```python
from build123d import *

# Parameters (mm, degrees)
SKETCH1_R               = 5.053
BASENUT_DEPTH           = 10.8
ENDCHAMFER_SIZE         = 0.947
ENDCHAMFER_SIZE2        = 0.546750705
ENDCHAMFER_PART_2_SIZE  = 0.947
ENDCHAMFER_PART_2_SIZE2 = 0.546750705


with BuildPart() as part:
    # Sketch1 → BaseNut (new body)
    with BuildSketch(Plane.XY):
        Polygon((10.392304845, 0), (5.196152423, 9), (-5.196152423, 9), (-10.392304845, 0), (-5.196152423, -9), (5.196152423, -9), align=None)
        Circle(SKETCH1_R, mode=Mode.SUBTRACT)
    extrude(amount=-BASENUT_DEPTH)

    # Sketch2 → Double-Chamfer (revolve, cut)
    with BuildSketch(Plane(origin=(0, 0, 0), x_dir=(1, 0, 0), z_dir=(0, 1, 0))):
        Polygon((-10.392304845, 10.8), (-8.625, 10.8), (-10.392304845, 9.779646072), align=None)
        Polygon((-10.392304845, 1.020353928), (-10.392304845, 0), (-8.625, 0), align=None)
    revolve(axis=Axis((0, 0, -3.375940562), (0, 0, 1)), mode=Mode.SUBTRACT)

    # EndChamfer
    endchamfer_edges = [part.edges().sort_by_distance(p)[0] for p in [
        (-5.053, 0, -10.8),
    ]]
    endchamfer_side = [part.faces().sort_by_distance(p)[0] for p in [
        (-5.053, 0, -5.4),
    ]]
    chamfer(endchamfer_edges, length=ENDCHAMFER_SIZE, length2=ENDCHAMFER_SIZE2, reference=endchamfer_side[0])

    # EndChamfer part 2
    endchamfer_part_2_edges = [part.edges().sort_by_distance(p)[0] for p in [
        (-5.053, 0, 0),
    ]]
    endchamfer_part_2_side = [part.faces().sort_by_distance(p)[0] for p in [
        (8.38104816, 0, 0),
    ]]
    chamfer(endchamfer_part_2_edges, length=ENDCHAMFER_PART_2_SIZE, length2=ENDCHAMFER_PART_2_SIZE2, reference=endchamfer_part_2_side[0])


solid = part.part
```
Part model, mm, in its own coordinate system. Round coordinates to 2 decimals unless told otherwise and drop trailing zeros. Write each loop counter-clockwise with the first axis right and the second up, starting at its lowest first coordinate (ties: lowest second). Pieces come first, ordered by that corner, then holes.
Item 1: Cut at A-A, the plane x = 0. Give the cut face in (y, z) (1 decimal), plus the area to 3 significant figures.
Results:
outline: (-9, -10.6) - (-8.6, -10.8) - (-5.6, -10.8) - (-5.1, -9.9) - (-5.1, -0.5) - (-6, 0) - (-8.6, 0) - (-9, -0.2) - close; (5.1, -9.9) - (5.6, -10.8) - (8.6, -10.8) - (9, -10.6) - (9, -0.2) - (8.6, 0) - (6, 0) - (5.1, -0.5) - close
area: 84.1 mm2
Item 2: Probe L1, parallel to Y at x = 0, z = -7.5; L2, parallel to X at y = 4, z = -8.25; L3, parallel to Y at x = 3.25, z = -6.5. List the from-to ranges inside material, lowest first.
Results:
L1: y = -9 to -5.05, 5.05 to 9
L2: x = -8.08 to -3.09, 3.09 to 8.08
L3: y = -9 to -3.87, 3.87 to 9
Item 3: Drop a flat-ended pin along its axis: pin 1 Ø1.5 at (x, z) = (7, -2) entering from +Y. Give the stop position or say it passes through.
Results:
pin 1: stops at y = 7.17
Item 4: Two-plate mould, pull along Y, no slides. Class faces 1 (the cylindrical face through (-4.01, -3.075, -5.135)), 2 (the flat face through (7.83, 4.44, -5.33)), 3 (the flat face through (0, -9, -5)): +Y half, -Y half, draft (parallel to the pull), parting line (faces both ways), or undercut.
Results:
face 1: undercut
face 2: +Y half
face 3: -Y half
